For this review, take the finished solid that the model builds, in its own axes (mm). A direction names the side the tool comes from. Coordinates: 2 decimals unless noted, no trailing zeros. Loops run counter-clockwise (first coordinate to the right, second up) from the corner with the lowest first, then second, coordinate; pieces in that order, holes last. Notation, with made-up numbers: (65.5, 42) -> (73.5, 42) arc R24 cw to (73.5, 76) -> close; hole circle Ø4 at (65, 41). An arc over 180 degrees is marked (long way). Use a Markdown table: item, result.
Autodesk Inventor part; units mm, degrees
ref_plane "Work Plane1" through (-24.73, 0, 10) normal (0, 0, 1) x (1, 0, 0)
ref_plane "YZ Plane" through (0, 0, 0) normal (1, 0, 0) x (0, 1, 0)
ref_plane "XZ Plane" through (0, 0, 0) normal (0, 1, 0) x (-1, 0, 0)
sketch "Sketch1" plane through (0, 0, 0) normal (0, 1, 0) x (-1, 0, 0)
  line L0 (0, 0) -> (40, 0)
  line L1 (40, 0) -> (40, 20)
  line L2 (40, 20) -> (0, 20)
  line L3 (0, 20) -> (0, 0)
  line L4 (0, 14) -> (4, 14)
  line L5 (4, 14) -> (4, 6)
  line L6 (4, 6) -> (0, 6)
  line L7 (0, 6) -> (0, 14)
  line L8 (40, 14) -> (36, 14)
  line L9 (36, 14) -> (36, 6)
  line L10 (36, 6) -> (40, 6)
  line L11 (40, 6) -> (40, 14)
  line L12 (6, 0) -> (14, 0)
  line L13 (14, 0) -> (14, 4)
  line L14 (14, 4) -> (6, 4)
  line L15 (6, 4) -> (6, 0)
  line L16 (26, 0) -> (34, 0)
  line L17 (34, 0) -> (34, 4)
  line L18 (34, 4) -> (26, 4)
  line L19 (26, 4) -> (26, 0)
  line L20 (6, 20) -> (14, 20)
  line L21 (14, 20) -> (14, 16)
  line L22 (14, 16) -> (6, 16)
  line L23 (6, 16) -> (6, 20)
  line L24 (26, 20) -> (34, 20)
  line L25 (34, 20) -> (34, 16)
  line L26 (34, 16) -> (26, 16)
  line L27 (26, 16) -> (26, 20)
  dimension "d0" = 40
  dimension "d1" = 20
  dimension "d2" = 6
  dimension "d3" = 8
  dimension "d4" = 4
  dimension "d5" = 8
  dimension "d6" = 6
  dimension "d7" = 4
  dimension "d8" = 4
  dimension "d9" = 8
  dimension "d10" = 6
  dimension "d11" = 4
extrude "Extrusion1" add sketch "Sketch1" along normal blind 413.004 contours L3 L6 L5 L4 L2 L23 L22 L21 L27 L26 L25 L1 L8 L9 L10 L0 L17 L18 L19 L13 L14 L15
fillet "Fillet1" radius 1.27 16 edges at (-40, 206.502, 20) (-40, 206.502, 14) (-40, 206.502, 6) (-40, 206.502, 0) (-34, 206.502, 0) (-34, 206.502, 20) (-26, 206.502, 20) (-14, 206.502, 20) (-6, 206.502, 20) (0, 206.502, 20) (0, 206.502, 14) (0, 206.502, 6) (0, 206.502, 0) (-6, 206.502, 0) (-14, 206.502, 0) (-26, 206.502, 0)
ref_plane "Work Plane1" through (-24.73, 0, 10) normal (0, 0, 1) x (1, 0, 0)
properties part number "20X40long" material "Aluminum 6061"
(1) For pin 1 Ø6.5 at (x, y) = (-31, 124) entering from +Z; pin 2 Ø5 at (x, z) = (-29.5, 4.5) entering from -Y; pin 3 Ø1.5 at (y, z) = (229, 14) entering from +X; pin 4 Ø4 at (y, z) = (139.5, 9.5) entering from -X, all flat-tipped, find the tip position at first contact; note any pin that passes through.
Found:
| item | result |
|---|---|
| pin 1 | stops at z = 19.49 |
| pin 2 | stops at y = 0 |
| pin 3 | stops at x = -0.11 |
| pin 4 | stops at x = -36 |
(2) Mouldability with a two-part tool opening along X and no side actions: class faces 1 (the face through (-36, 204, 10)), 2 (the face through (-20, 0, 10)), 3 (the face through (-30, 204, 16)) as pulls with the +X half, pulls with the -X half, needs draft (parallel to the pull), parting line crosses it, or undercut.
Found:
| item | result |
|---|---|
| face 1 | pulls with the -X half |
| face 2 | needs draft |
| face 3 | undercut |
(3) For line 1 along X through (y, z) = (215.5, 2.5); line 2 along Z through (x, y) = (-37.5, 74); line 3 along Z through (x, y) = (-30.5, 206), list the stretches that pass through material, from the lowest coordinate up.
Found:
| item | result |
|---|---|
| line 1 | x = -40 to -34, -26 to -14, -6 to 0 |
| line 2 | z = 0 to 6, 14 to 20 |
| line 3 | z = 4 to 16 |
(4) Take a section at A-A on x = -30.5. Write out the cut boundary in (y, z).
Found:
| item | result |
|---|---|
| outline | (0, 4) -> (413, 4) -> (413, 16) -> (0, 16) -> close |
(5) For faces 4 (the face through (-4, 204, 10)), 5 (the face through (-10, 204, 16)), 6 (the face through (-30, 204, 4)), list the 3-axis set-ups (+Z, -Z, +X, -X, +Y, -Y) from which the entire face can be reached by the end or side of a thin tool; tool diameter is ignored.
Found:
| item | result |
|---|---|
| face 4 | +X, +Y, -Y |
| face 5 | +Z, +Y, -Y |
| face 6 | -Z, +Y, -Y |
